from build123d import *

# Parameters (mm, degrees)
SKETCH1_W            = 72.3
SKETCH1_H            = 56.5
SKETCH1_W_2          = 52.3
SKETCH1_H_2          = 36.5
BOSS_EXTRUDE1_DEPTH  = 3.3
SKETCH2_W            = 72.3
SKETCH2_H            = 2
BOSS_EXTRUDE2_DEPTH  = 45
SKETCH3_W            = 2
SKETCH3_H            = 45
BOSS_EXTRUDE3_DEPTH  = 54.5
SKETCH5_W            = 72.3
SKETCH5_H            = 56.5
SKETCH5_W_2          = 43.2
SKETCH5_H_2          = 33.3
BOSS_EXTRUDE6_DEPTH  = 0.8
SKETCH6_W            = 68.3
SKETCH6_H            = 1.5
BOSS_EXTRUDE7_DEPTH  = 7.8
BOSS_EXTRUDE8_DEPTH  = 7.8
SKETCH8_W            = 18.0427139
SKETCH8_H            = 6
SKETCH8_W_2          = 15
SKETCH8_H_2          = 3
BOSS_EXTRUDE9_DEPTH  = 10
SKETCH9_W            = 4
SKETCH9_H            = 26.5
CUT_EXTRUDE1_DEPTH   = 2
SKETCH10_W           = 2
SKETCH10_H           = 30
CUT_EXTRUDE2_DEPTH   = 40
SKETCH11_W           = 2
SKETCH11_H           = 1
BOSS_EXTRUDE10_DEPTH = 20
SKETCH13_W           = 15
SKETCH13_H           = 3
BOSS_EXTRUDE11_DEPTH = 5
SKETCH12_W           = 6.2
SKETCH12_H           = 6.2
CUT_EXTRUDE3_DEPTH   = 10
SKETCH14_W           = 18.0427139
SKETCH14_H           = 5
CUT_EXTRUDE4_DEPTH   = 25
SKETCH15_W           = 29.613072231
SKETCH15_H           = 15.101269166
CUT_EXTRUDE5_DEPTH   = 2
SKETCH17_W           = 5.5
SKETCH17_H           = 8
BOSS_EXTRUDE12_DEPTH = 6
SKETCH20_W           = 2
SKETCH20_H           = 3
BOSS_EXTRUDE14_DEPTH = 43
SKETCH21_R           = 14.5
BOSS_EXTRUDE15_DEPTH = 8
SKETCH22_R           = 12.75
CUT_EXTRUDE6_DEPTH   = 6
FILLET1_R            = 2
SKETCH23_W           = 17.408302374
SKETCH23_H           = 1
BOSS_EXTRUDE16_DEPTH = 2
BOSS_EXTRUDE17_REACH = 131.062
SKETCH24_W           = 1.408302374
SKETCH24_H           = 2
SKETCH24_W_2         = 1.408302375
SKETCH25_W           = 17.4
SKETCH25_H           = 2
BOSS_EXTRUDE18_DEPTH = 2
SKETCH26_W           = 6.4
SKETCH26_H           = 6.4
CUT_EXTRUDE7_DEPTH   = 4.1
SKETCH28_W           = 5
SKETCH28_H           = 3
CUT_EXTRUDE9_DEPTH   = 2
SKETCH29_R           = 14.5
SKETCH29_R_2         = 12.75
CUT_EXTRUDE10_DEPTH  = 3
FILLET2_R            = 10


with BuildPart() as part:
    # Sketch1 → Boss-Extrude1 (new body)
    with BuildSketch(Plane(origin=(0, 0, 0), x_dir=(1, 0, 0), z_dir=(0, 1, 0))):
        with Locations((59.895731411, 31.047033621)):
            Rectangle(SKETCH1_W, SKETCH1_H)
        with Locations((59.895731411, 31.047033621)):
            Rectangle(SKETCH1_W_2, SKETCH1_H_2, mode=Mode.SUBTRACT)
    extrude(amount=BOSS_EXTRUDE1_DEPTH)

    # Sketch2 → Boss-Extrude2 (add)
    with BuildSketch(Plane.XZ):
        with Locations((59.895731411, -3.797033621)):
            Rectangle(SKETCH2_W, SKETCH2_H)
    extrude(amount=BOSS_EXTRUDE2_DEPTH)

    # Sketch3 → Boss-Extrude3 (add)
    with BuildSketch(Plane(origin=(0, 0, -4.797033621), x_dir=(-1, 0, 0), z_dir=(0, 0, -1))):
        with Locations((-95.045731411, -22.5)):
            Rectangle(SKETCH3_W, SKETCH3_H)
        with Locations((-24.745731411, -22.5)):
            Rectangle(SKETCH3_W, SKETCH3_H)
    extrude(amount=BOSS_EXTRUDE3_DEPTH)

    # Sketch5 → Boss-Extrude6 (add)
    with BuildSketch(Plane(origin=(0, 3.3, 0), x_dir=(1, 0, 0), z_dir=(0, 1, 0))):
        with Locations((59.895731411, 31.047033621)):
            Rectangle(SKETCH5_W, SKETCH5_H)
        with Locations((62.845731411, 31.047033621)):
            Rectangle(SKETCH5_W_2, SKETCH5_H_2, mode=Mode.SUBTRACT)
    extrude(amount=BOSS_EXTRUDE6_DEPTH)

    # Sketch6 → Boss-Extrude7 (add)
    with BuildSketch(Plane(origin=(0, 0, -4.797033621), x_dir=(-1, 0, 0), z_dir=(0, 0, -1))):
        with Locations((-59.895731411, -0.75)):
            Rectangle(SKETCH6_W, SKETCH6_H)
    extrude(amount=BOSS_EXTRUDE7_DEPTH)

    # Sketch7 → Boss-Extrude8 (add)
    with BuildSketch(Plane(origin=(0, 0, -4.797033621), x_dir=(-1, 0, 0), z_dir=(0, 0, -1))):
        Polygon((-87.045731411, -1.5), (-87.045731411, -4.5), (-72.045731411, -4.5), (-72.045731411, -1.5), (-70.545731411, -1.5), (-70.545731411, -6), (-88.545731411, -6), (-88.545731411, -1.5), align=None)
    extrude(amount=BOSS_EXTRUDE8_DEPTH)

    # Sketch8 → Boss-Extrude9 (add)
    with BuildSketch(Plane(origin=(0, 0, -59.297033621), x_dir=(-1, 0, 0), z_dir=(0, 0, -1))):
        with Locations((-79.524374461, -3)):
            Rectangle(SKETCH8_W, SKETCH8_H)
        with Locations((-79.545731411, -3)):
            Rectangle(SKETCH8_W_2, SKETCH8_H_2, mode=Mode.SUBTRACT)
    extrude(amount=-BOSS_EXTRUDE9_DEPTH)

    # Sketch9 → Cut-Extrude1 (cut)
    with BuildSketch(Plane.XZ):
        with Locations((88.045731411, -31.047033621)):
            Rectangle(SKETCH9_W, SKETCH9_H)
    extrude(amount=-CUT_EXTRUDE1_DEPTH, mode=Mode.SUBTRACT)

    # Sketch10 → Cut-Extrude2 (cut)
    with BuildSketch(Plane(origin=(0, 0, -59.297033621), x_dir=(-1, 0, 0), z_dir=(0, 0, -1))):
        with Locations((-95.045731411, -30)):
            Rectangle(SKETCH10_W, SKETCH10_H)
    extrude(amount=-CUT_EXTRUDE2_DEPTH, mode=Mode.SUBTRACT)

    # Sketch11 → Boss-Extrude10 (add)
    with BuildSketch(Plane.XZ.offset(1.5)):
        with Locations((93.045731411, -7.697033621)):
            Rectangle(SKETCH11_W, SKETCH11_H)
        with Locations((26.745731411, -7.697033621)):
            Rectangle(SKETCH11_W, SKETCH11_H)
    extrude(amount=BOSS_EXTRUDE10_DEPTH)

    # Sketch13 → Boss-Extrude11 (add)
    with BuildSketch(Plane(origin=(0, 0, -59.297033621), x_dir=(-1, 0, 0), z_dir=(0, 0, -1))):
        Polygon((-96.045731411, 4.1), (-96.045731411, -15), (-94.045731411, -15), (-94.045731411, 0), (-88.545731411, 0), (-88.545731411, -6), (-70.503017511, -6), (-70.503017511, 0), (-25.745731411, 0), (-25.745731411, -45), (-23.745731411, -45), (-23.745731411, 4.1), align=None)
        with Locations((-79.545731411, -3)):
            Rectangle(SKETCH13_W, SKETCH13_H, mode=Mode.SUBTRACT)
    extrude(amount=BOSS_EXTRUDE11_DEPTH)

    # Sketch12 → Cut-Extrude3 (cut)
    with BuildSketch(Plane(origin=(0, 4.1, 0), x_dir=(1, 0, 0), z_dir=(0, 1, 0))):
        with Locations((42.845731411, 57.197033621)):
            Rectangle(SKETCH12_W, SKETCH12_H)
        with Locations((54.045731411, 57.197033621)):
            Rectangle(SKETCH12_W, SKETCH12_H)
    extrude(amount=-CUT_EXTRUDE3_DEPTH, mode=Mode.SUBTRACT)

    # Sketch14 → Cut-Extrude4 (cut)
    with BuildSketch(Plane.XZ):
        with Locations((79.524374461, -51.797033621)):
            Rectangle(SKETCH14_W, SKETCH14_H)
    extrude(amount=CUT_EXTRUDE4_DEPTH, mode=Mode.SUBTRACT)

    # Sketch15 → Cut-Extrude5 (cut)
    with BuildSketch(Plane(origin=(0, 0, -64.297033621), x_dir=(-1, 0, 0), z_dir=(0, 0, -1))):
        with Locations((-85.309553627, -7.550634583)):
            Rectangle(SKETCH15_W, SKETCH15_H)
    extrude(amount=-CUT_EXTRUDE5_DEPTH, mode=Mode.SUBTRACT)

    # Sketch17 → Boss-Extrude12 (add)
    with BuildSketch(Plane.XZ):
        with Locations((91.295731411, -58.297033621)):
            Rectangle(SKETCH17_W, SKETCH17_H)
    extrude(amount=BOSS_EXTRUDE12_DEPTH)

    # Sketch20 → Boss-Extrude14 (add)
    with BuildSketch(Plane(origin=(0, 0, -19.297033621), x_dir=(-1, 0, 0), z_dir=(0, 0, -1))):
        with Locations((-95.045731411, -16.5)):
            Rectangle(SKETCH20_W, SKETCH20_H)
    extrude(amount=BOSS_EXTRUDE14_DEPTH)

    # Sketch21 → Boss-Extrude15 (add)
    with BuildSketch(Plane(origin=(0, 0, -62.297033621), x_dir=(-1, 0, 0), z_dir=(0, 0, -1))):
        with Locations((-95.045731411, -18)):
            Circle(SKETCH21_R)
    extrude(amount=-BOSS_EXTRUDE15_DEPTH)

    # Sketch22 → Cut-Extrude6 (cut)
    with BuildSketch(Plane(origin=(0, 0, -62.297033621), x_dir=(-1, 0, 0), z_dir=(0, 0, -1))):
        with Locations((-95.045731411, -18)):
            Circle(SKETCH22_R)
    extrude(amount=-CUT_EXTRUDE6_DEPTH, mode=Mode.SUBTRACT)

    # Fillet1
    fillet1_edges = [part.edges().sort_by_distance(p)[0] for p in [
        (94.045731411, -9, -54.297033621),
        (95.045731411, -18, -54.297033621),
        (96.045731411, -10.767261929, -54.297033621),
    ]]
    fillet(fillet1_edges, radius=FILLET1_R)

    # Sketch23 → Boss-Extrude16 (add)
    with BuildSketch(Plane.XZ):
        with Locations((48.449882598, -53.597033621)):
            Rectangle(SKETCH23_W, SKETCH23_H)
    extrude(amount=BOSS_EXTRUDE16_DEPTH)

    # Boss-Extrude17: up to this face of the body (flat: up to its plane)
    boss_extrude17_end = Plane(part.part.faces().sort_by_distance((83.274374461, -0.50799444, -62.297033621))[0])
    # Sketch24 → Boss-Extrude17 (add, up to the picked face)
    with BuildSketch(Plane(origin=(0, 0, -54.097033621), x_dir=(-1, 0, 0), z_dir=(0, 0, -1)), mode=Mode.PRIVATE) as boss_extrude17_sk1:
        with Locations((-54.049882598, -1)):
            Rectangle(SKETCH24_W, SKETCH24_H)
    boss_extrude17_tool1 = split(extrude(boss_extrude17_sk1.sketch, amount=BOSS_EXTRUDE17_REACH, mode=Mode.PRIVATE), bisect_by=boss_extrude17_end, keep=Keep.BOTH, mode=Mode.PRIVATE)
    # Sketch24 → Boss-Extrude17 (add, up to the picked face)
    with BuildSketch(Plane(origin=(0, 0, -54.097033621), x_dir=(-1, 0, 0), z_dir=(0, 0, -1)), mode=Mode.PRIVATE) as boss_extrude17_sk2:
        with Locations((-42.841580224, -1)):
            Rectangle(SKETCH24_W_2, SKETCH24_H)
    boss_extrude17_tool2 = split(extrude(boss_extrude17_sk2.sketch, amount=BOSS_EXTRUDE17_REACH, mode=Mode.PRIVATE), bisect_by=boss_extrude17_end, keep=Keep.BOTH, mode=Mode.PRIVATE)
    add(boss_extrude17_tool1.solids().sort_by(Axis((54.049883, -1, -54.097034), (0, 0, -1)))[0])
    add(boss_extrude17_tool2.solids().sort_by(Axis((42.84158, -1, -54.097034), (0, 0, -1)))[0])

    # Sketch25 → Boss-Extrude18 (add)
    with BuildSketch(Plane.XZ):
        with Locations((48.445731411, -61.297033621)):
            Rectangle(SKETCH25_W, SKETCH25_H)
    extrude(amount=BOSS_EXTRUDE18_DEPTH)

    # Sketch26 → Cut-Extrude7 (cut)
    with BuildSketch(Plane(origin=(0, 4.1, 0), x_dir=(1, 0, 0), z_dir=(0, 1, 0))):
        with Locations((42.845731411, 57.197033621)):
            Rectangle(SKETCH26_W, SKETCH26_H)
        with Locations((54.045731411, 57.197033621)):
            Rectangle(SKETCH26_W, SKETCH26_H)
    extrude(amount=-CUT_EXTRUDE7_DEPTH, mode=Mode.SUBTRACT)

    # Sketch28 → Cut-Extrude9 (cut)
    with BuildSketch(Plane(origin=(0, 0, -4.797033621), x_dir=(-1, 0, 0), z_dir=(0, 0, -1))):
        with Locations((-84.545731411, -3)):
            Rectangle(SKETCH28_W, SKETCH28_H)
        with Locations((-74.545731411, -3)):
            Rectangle(SKETCH28_W, SKETCH28_H)
    extrude(amount=-CUT_EXTRUDE9_DEPTH, mode=Mode.SUBTRACT)

    # Sketch29 → Cut-Extrude10 (cut)
    with BuildSketch(Plane(origin=(0, 0, -62.297033621), x_dir=(-1, 0, 0), z_dir=(0, 0, -1))):
        with Locations((-95.045731411, -18)):
            Circle(SKETCH29_R)
        with Locations((-95.045731411, -18)):
            Circle(SKETCH29_R_2, mode=Mode.SUBTRACT)
    extrude(amount=-CUT_EXTRUDE10_DEPTH, mode=Mode.SUBTRACT)

    # Fillet2
    fillet2_edges = [part.edges().sort_by_distance(p)[0] for p in [
        (96.045731411, -3.534523859, -55.797033621),
    ]]
    fillet(fillet2_edges, radius=FILLET2_R)


solid = part.part
Build history of the part. All positions in model axes, mm. A direction names the side the tool comes from. Coordinates: 2 decimals unless noted, no trailing zeros. Order: outer loops, then holes, each group sorted by start corner. A loop starts at its lowest first (then second) coordinate and runs counter-clockwise, first axis right, second up. Notation, with made-up numbers: (-16, 15.5) - (29, 15.5) arc R25 cw to (29, 52.5) - close; hole circle Ø3 at (67, 86.25). An arc over 180 degrees is marked (long way). Write item = value, one per line. Start each with the question number.
1) Saw through at D-D on y = -37.5. Write the cut outline in (x, z).
2) Saw through at C-C on y = -25. Write the cut outline in (x, z), then the cut area to 3 significant figures.
3) Flat gauge pins, fed straight in: pin 1 Ø4 at (x, z) = (39.5, -42.5) entering from -Y; pin 2 Ø0.5 at (y, z) = (-13, -7.5) entering from +X; pin 3 Ø1.5 at (x, y) = (85.5, -32.5) entering from -Z. Where does each tip first touch, or does it go through?
4) Saw through at A-A on x = 74.5. Write the cut outline in (y, z).
5) 3-axis set-ups, long thin cutter, end or side, ignore diameter. For faces 5 (the face through (79, -6, -58)), 6 (the face through (82.046, -3, -4)), 7 (the face through (60, 2, -12.797)): which of +Z, -Z, +X, -X, +Y, -Y reach the whole face in a straight line?
6) Two-plate mould, pull along Z, no slides. Class faces 1 (the face through (59, -21, -2.797)), 2 (the face through (90, -16, -54.297)), 3 (the face through (56, -1, -60.297)), 4 (the face through (77.046, -3, -4)): pulls with the +Z half, pulls with the -Z half, needs draft (parallel to the pull), parting line crosses it, or undercut.
7) Saw through at B-B on z = -36. Write the cut outline in (x, y).
8) Wall check: line 1 along X through (y, z) = (-17, -21); line 2 along Z through (x, y) = (91, -22); line 3 along Z through (x, y) = (53, -27). Give the ranges that are in metal, low to high. Write a range as from..to.
From the geometry:
q1.outline = (23.75, -64.3) - (25.75, -64.3) - (25.75, -4.8) - (94.05, -4.8) - (94.05, -19.3) - (96.05, -19.3) - (96.05, -2.8) - (23.75, -2.8) - close
q2.outline = (23.75, -64.3) - (25.75, -64.3) - (25.75, -4.8) - (94.05, -4.8) - (94.05, -19.3) - (96.05, -19.3) - (96.05, -2.8) - (23.75, -2.8) - close; (82.35, -59.3) - (84.39, -59.3) - (84.39, -56.3) - (105.7, -56.3) - (105.7, -59.3) - (107.74, -59.3) - (107.74, -54.3) - (82.35, -54.3) - close
q2.area = 356 mm^2
q3.pin_1 = 3.3
q3.pin_2 = 96.05
q3.pin_3 = -4.8
q4.outline = (-45, -4.8) - (-6, -4.8) - (-6, -12.6) - (-4.5, -12.6) - (-4.5, -2.8) - (-45, -2.8) - close; (-6, -62.3) - (-4.5, -62.3) - (-4.5, -54.3) - (-6, -54.3) - close; (-1.5, -62.3) - (0, -62.3) - (0, -64.3) - (4.1, -64.3) - (4.1, -47.7) - (3.3, -47.7) - (3.3, -49.3) - (0, -49.3) - (0, -54.3) - (-1.5, -54.3) - close; (-1.5, -12.6) - (0, -12.6) - (0, -12.8) - (3.3, -12.8) - (3.3, -14.4) - (4.1, -14.4) - (4.1, -2.8) - (-1.5, -2.8) - close
q5.face_5 = -Z
q5.face_6 = +Z, -Z
q5.face_7 = -Y
q6.face_1 = pulls with the +Z half
q6.face_2 = undercut
q6.face_3 = undercut
q6.face_4 = needs draft
q7.outline = (23.75, -45) - (25.75, -45) - (25.75, 0) - (33.75, 0) - (33.75, 3.3) - (41.25, 3.3) - (41.25, 4.1) - (23.75, 4.1) - close; (84.45, 3.3) - (86.05, 3.3) - (86.05, 2) - (90.05, 2) - (90.05, 0) - (94.05, 0) - (94.05, -18) - (96.05, -18) - (96.05, 4.1) - (84.45, 4.1) - close
q8.line_1 = 23.75..25.75, 94.05..96.05
q8.line_2 = -56.3..-54.3, -4.8..-2.8
q8.line_3 = -4.8..-2.8
